```python
from build123d import *

# Parameters (mm, degrees)
SKETCH1_W                = 50
SKETCH1_H                = 30
BOSS_EXTRUDE1_DEPTH      = 5
BOSS_EXTRUDE2_DEPTH      = 5
BOSS_EXTRUDE2_DEPTH_BACK = 5
SKETCH3_W                = 24
SKETCH3_H                = 25
CUT_EXTRUDE1_DEPTH       = 10
SKETCH4_R                = 2.5
CUT_EXTRUDE2_DEPTH       = 10
SKETCH5_R                = 2.5
CUT_EXTRUDE3_DEPTH       = 10


with BuildPart() as part:
    # Sketch1 → Boss-Extrude1 (new body)
    with BuildSketch(Plane.XY):
        Rectangle(SKETCH1_W, SKETCH1_H)
    extrude(amount=BOSS_EXTRUDE1_DEPTH)

    # Sketch2 → Boss-Extrude2 (add, two sides: drawn at the far end of the back side and taken through both)
    with BuildSketch(Plane(origin=(0, 0, 0), x_dir=(1, 0, 0), z_dir=(0, 1, 0)).offset(-BOSS_EXTRUDE2_DEPTH_BACK)):
        Polygon((-6.250199949, 30), (-6.250199949, 0), (6.250199949, 0), (6.250199949, 30), (16.958872349, 30), (16.958872349, 70), (-16.958872349, 70), (-16.958872349, 30), align=None)
    extrude(amount=BOSS_EXTRUDE2_DEPTH + BOSS_EXTRUDE2_DEPTH_BACK)

    # Sketch3 → Cut-Extrude1 (cut)
    with BuildSketch(Plane(origin=(0, 5, 0), x_dir=(1, 0, 0), z_dir=(0, 1, 0))):
        with Locations((-0.041127651, 50)):
            Rectangle(SKETCH3_W, SKETCH3_H)
    extrude(amount=-CUT_EXTRUDE1_DEPTH, mode=Mode.SUBTRACT)

    # Sketch4 → Cut-Extrude2 (cut)
    with BuildSketch(Plane(origin=(0, 0, 0), x_dir=(-1, 0, 0), z_dir=(0, 0, -1))):
        with Locations((-19.020005018, 9.402240441)):
            Circle(SKETCH4_R)
    extrude(amount=-CUT_EXTRUDE2_DEPTH, mode=Mode.SUBTRACT)

    # Sketch5 → Cut-Extrude3 (cut)
    with BuildSketch(Plane(origin=(0, 0, 0), x_dir=(-1, 0, 0), z_dir=(0, 0, -1))):
        with Locations((19.72045846, -8.8634301)):
            Circle(SKETCH5_R)
    extrude(amount=-CUT_EXTRUDE3_DEPTH, mode=Mode.SUBTRACT)


solid = part.part
```
Geometry check sheet. Reference: the model listing, model coordinates, mm. A direction names the side the tool comes from. Round coordinates to 2 decimals unless told otherwise and drop trailing zeros. Order: outer loops, then holes, each group sorted by start corner. A loop starts at its lowest first (then second) coordinate and runs counter-clockwise, first axis right, second up. Notation, with made-up numbers: (63.5, -30.75) - (69.5, -30.75) arc R24 cw to (69.5, 1.25) - close; hole circle Ø10 at (27.25, -22). An arc over 180 degrees is marked (long way). Use a Markdown table: item, result. Add a question column.
1) Mould release check, pull along Z, two halves, no side actions. Record for faces 1 (the cylindrical face through (17.866, 7.184, 2.465)), 2 (the flat face through (0, 0, -37.5)), 3 (the flat face through (0, 0, 5)), 4 (the flat face through (0, 0, -70)): released by +Z, released by -Z, zero draft, split by the parting line, or undercut.
2) Thickness scan on line 1 along Z through (x, y) = (8.5, -0.5); line 2 along Z through (x, y) = (-5.5, 0); line 3 along X through (y, z) = (3.75, -9). Record the ranges inside material, lowest first.
3) Gauge pin test, flat ends, axial feed: P1, Ø4.5, axis at x = 19.02, y = 9.4, coming from the +Z side; P2, Ø2, axis at y = 2, z = -23.5, coming from the +X side; P3, Ø11, axis at y = 1.5, z = -53, coming from the +X side; P4, Ø1.5, axis at x = 0, z = -36, coming from the -Y side. Record the tip position at first contact, or that the pin passes through.
4) Section check D-D (y = 11). Record the cut outline in (x, z).
5) Section check B-B (z = -47). Record the cut outline in (x, y), then the cut area to 3 significant figures.
6) Section check C-C (y = 2). Record the cut outline in (x, z), then the cut area to 3 significant figures.
7) Section check A-A (x = 1). Record the cut outline in (y, z).
8) Set-up check for faces 5 (the flat face through (0, 7, 0)), 6 (the flat face through (0, 5, -35)), 7 (the flat face through (16.959, 0, -50)), 8 (the flat face through (-16.959, 0, -50)), 9 (the flat face through (-12, 0, -30)): record each of +Z, -Z, +X, -X, +Y, -Y from which the full face is reachable in a straight line by a thin tool's end or side.
Established:
| question | item | result |
|---|---|---|
| 1 | face 1 | zero draft |
| 1 | face 2 | undercut |
| 1 | face 3 | released by +Z |
| 1 | face 4 | released by -Z |
| 2 | line 1 | -70 to -62.5, -37.5 to -30, 0 to 5 |
| 2 | line 2 | -70 to -62.5, -37.5 to 5 |
| 2 | line 3 | -6.25 to 6.25 |
| 3 | P1 | through |
| 3 | P2 | x = 6.25 |
| 3 | P3 | x = 16.96 |
| 3 | P4 | y = -5 |
| 4 | outline | (-25, 0) - (17.1, 0) - (17.1, 5) - (-25, 5) - close; (20.94, 0) - (25, 0) - (25, 5) - (20.94, 5) - close |
| 5 | outline | (-16.96, -5) - (-12.04, -5) - (-12.04, 5) - (-16.96, 5) - close; (11.96, -5) - (16.96, -5) - (16.96, 5) - (11.96, 5) - close |
| 5 | area | 99.2 mm2 |
| 6 | outline | (-25, 0) - (-6.25, 0) - (-6.25, -30) - (-16.96, -30) - (-16.96, -70) - (16.96, -70) - (16.96, -30) - (6.25, -30) - (6.25, 0) - (25, 0) - (25, 5) - (-25, 5) - close; hole (-12.04, -62.5) - (11.96, -62.5) - (11.96, -37.5) - (-12.04, -37.5) - close |
| 6 | area | 1,380 mm2 |
| 7 | outline | (-15, 0) - (-5, 0) - (-5, -37.5) - (5, -37.5) - (5, 0) - (15, 0) - (15, 5) - (-15, 5) - close; (-5, -70) - (5, -70) - (5, -62.5) - (-5, -62.5) - close |
| 8 | face 5 | none |
| 8 | face 6 | -Z, +X, -X, +Y |
| 8 | face 7 | -Z, +X, +Y, -Y |
| 8 | face 8 | -Z, -X, +Y, -Y |
| 8 | face 9 | -X, +Y, -Y |
